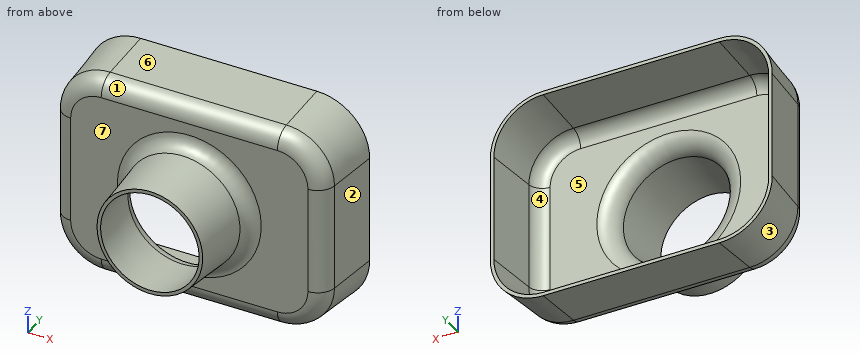
```python
from build123d import *

# Parameters (mm, degrees)
BOSS_EXTRUDE1_DEPTH = 25.4
BOSS_EXTRUDE1_DRAFT = -5
BOSS_EXTRUDE2_REACH = 83.32
SKETCH3_R           = 19.05
BOSS_EXTRUDE2_DRAFT = 5
FILLET1_R           = 5.08
FILLET2_R           = 6.35
SHELL1_T            = -1.27


with BuildPart() as part:
    # Sketch1 → Boss-Extrude1 (with draft: the straight prism first)
    with BuildSketch(Plane(origin=(0, 0, 0), x_dir=(1, 0, 0), z_dir=(0, 1, 0))):
        with BuildLine():
            ThreePointArc((31.75, -38.1), (45.220384182, -32.520384182), (50.8, -19.05))
            Line((50.8, -19.05), (50.8, 19.05))
            ThreePointArc((50.8, 19.05), (45.220384182, 32.520384182), (31.75, 38.1))
            Line((31.75, 38.1), (-31.75, 38.1))
            ThreePointArc((-31.75, 38.1), (-45.220384182, 32.520384182), (-50.8, 19.05))
            Line((-50.8, 19.05), (-50.8, -19.05))
            ThreePointArc((-50.8, -19.05), (-45.220384182, -32.520384182), (-31.75, -38.1))
            Line((-31.75, -38.1), (31.75, -38.1))
        make_face()
    extrude(amount=-BOSS_EXTRUDE1_DEPTH)
    # Boss-Extrude1: the draft: its side faces are tilted about the plane it starts from
    boss_extrude1_sides = [part.faces().sort_by_distance(p)[0] for p in [
        (45.220384182, -12.7, 32.520384182),
        (50.8, -12.7, 0),
        (45.220384182, -12.7, -32.520384182),
        (0, -12.7, -38.1),
        (-45.220384182, -12.7, -32.520384182),
        (-50.8, -12.7, 0),
        (-45.220384182, -12.7, 32.520384182),
        (0, -12.7, 38.1),
    ]]
    draft(boss_extrude1_sides, Plane(origin=(0, 0, 0), x_dir=(1, 0, 0), z_dir=(0, 1, 0)), BOSS_EXTRUDE1_DRAFT)




with BuildPart() as boss_extrude2_long_prism_1:
    # Sketch3 → Boss-Extrude2 (the long prism of profile 1, to be tilted and cut off)
    with BuildSketch(Plane(origin=(0, -50.8, 0), x_dir=(-1, 0, 0), z_dir=(0, -1, 0))):
        Circle(SKETCH3_R)
    extrude(amount=-BOSS_EXTRUDE2_REACH)
    boss_extrude2_tool1_sides = [boss_extrude2_long_prism_1.faces().sort_by_distance(p)[0] for p in [
        (19.05, -9.14, 0),
    ]]
    draft(boss_extrude2_tool1_sides, Plane(origin=(0, -50.8, 0), x_dir=(-1, 0, 0), z_dir=(0, -1, 0)), BOSS_EXTRUDE2_DRAFT)  # the draft: side faces tilted about the start plane


with BuildPart() as part_1:
    add(part.part)
    boss_extrude2_tool1 = boss_extrude2_long_prism_1.part - part.part
    add(boss_extrude2_tool1.solids().sort_by_distance((0, -50.8, 0))[0])

    # Fillet1
    fillet1_edges = [part_1.edges().sort_by_distance(p)[0] for p in [
        (21.272212054, -25.4, 0),
    ]]
    fillet(fillet1_edges, radius=FILLET1_R)

    # Fillet2
    fillet2_edges = [part_1.edges().sort_by_distance(p)[0] for p in [
        (-43.649042969, -25.4, 30.949042969),
        (0, -25.4, 35.877787946),
        (43.649042969, -25.4, 30.949042969),
        (48.577787946, -25.4, 0),
        (43.649042969, -25.4, -30.949042969),
        (0, -25.4, -35.877787946),
        (-43.649042969, -25.4, -30.949042969),
        (-48.577787946, -25.4, 0),
    ]]
    fillet(fillet2_edges, radius=FILLET2_R)

    # Shell1
    shell1_openings = [part_1.faces().sort_by_distance(p)[0] for p in [
        (0, -50.8, 0),
        (0, 0, 0),
    ]]
    offset(amount=SHELL1_T, openings=shell1_openings, kind=Kind.INTERSECTION)


solid = part_1.part
```
Input: part model. Units: mm. Frame: model coordinates. Face numbers are marked on the shaded views. A direction names the side the tool comes from. Give positions to 0.01 mm unless a question says otherwise; leave off trailing zeros. Order: outer loops, then holes, each group sorted by start corner. A loop starts at its lowest first (then second) coordinate and runs counter-clockwise, first axis right, second up. Notation, with made-up numbers: M -2.5,-33.75 L 1.5,-33.75 A33 cw 1.5,2.25 Z; hole C 0.5,88.25 d5. An arc over 180 degrees is marked long. Return JSON: item names as keys, results as strings.
Item 1: Ray query, probe 1 along X at (y, z) = (-21, -24.5); probe 2 along X at (y, z) = (-46, -1); probe 3 along Z at (x, y) = (-38.5, -3.5). Return the intervals inside material, ascending.
Solutions:
{"probe 1": "-47.91 to -46.47, 46.47 to 47.91", "probe 2": "-19.44 to -18.17, 18.17 to 19.44", "probe 3": "-36.54 to -35.16, 35.16 to 36.54"}
Item 2: Cut plane D-D (y = -16). Return loops of the section in (x, z).
Solutions:
{"outline": "M -49.4,-19.05 A17.65 ccw -31.75,-36.7 L 31.75,-36.7 A17.65 ccw 49.4,-19.05 L 49.4,19.05 A17.65 ccw 31.75,36.7 L -31.75,36.7 A17.65 ccw -49.4,19.05 Z; hole M -48.13,-19.05 A16.38 ccw -31.75,-35.43 L 31.75,-35.43 A16.38 ccw 48.13,-19.05 L 48.13,19.05 A16.38 ccw 31.75,35.43 L -31.75,35.43 A16.38 ccw -48.13,19.05 Z"}
Item 3: Pull-direction query (X, two-part tool) for the marked faces 1, 2, 3 and 4; classes: +X half, -X half, draft (parallel to the pull), parting line (faces both ways), or undercut.
Solutions:
{"face 1": "draft", "face 2": "+X half", "face 3": "-X half", "face 4": "undercut"}
Item 4: First-contact query: P1, Ø10, axis at x = -11, y = -21.5, coming from the +Z side; P2, Ø6, axis at x = 30.5, z = -18.5, coming from the +Y side; P3, Ø10, axis at x = -31, y = -5.5, coming from the +Z side. Flat tips, straight axial feed; report the tip coordinate or a pass-through.
Solutions:
{"P1": "z = 36.66", "P2": "y = -24.13", "P3": "z = 38.06"}
Item 5: Access query for the marked faces 5, 6 and 7. Directions: +Z, -Z, +X, -X, +Y, -Y. A direction counts if a zero-diameter tool reaches every point of the face in a straight line with its end or side. Return the directions, or none.
Solutions:
{"face 5": "+Y", "face 6": "+Z, +X, -X, -Y", "face 7": "-Y"}
Item 6: Cut plane C-C (x = 0). Return loops of the section in (y, z).
Solutions:
{"outline": "M -50.8,-19.05 L -30.04,-20.87 A5.08 cw -25.4,-25.93 L -25.4,-30.06 A6.35 ccw -19.6,-36.38 L 0,-38.1 L 0,-36.83 L -19.49,-35.12 A5.08 cw -24.13,-30.06 L -24.13,-25.93 A6.35 ccw -29.93,-19.6 L -50.8,-17.78 Z; M -50.8,17.78 L -29.93,19.6 A6.35 ccw -24.13,25.93 L -24.13,30.06 A5.08 cw -19.49,35.12 L 0,36.83 L 0,38.1 L -19.6,36.38 A6.35 ccw -25.4,30.06 L -25.4,25.93 A5.08 cw -30.04,20.87 L -50.8,19.05 Z"}
Item 7: Cut plane A-A (z = 0). Return loops of the section in (x, y).
Solutions:
{"outline": "M -50.8,0 L -49.08,-19.6 A6.35 ccw -42.76,-25.4 L -25.93,-25.4 A5.08 cw -20.87,-30.04 L -19.05,-50.8 L -17.78,-50.8 L -19.6,-29.93 A6.35 ccw -25.93,-24.13 L -42.76,-24.13 A5.08 cw -47.82,-19.49 L -49.53,0 Z; M 17.78,-50.8 L 19.05,-50.8 L 20.87,-30.04 A5.08 cw 25.93,-25.4 L 42.76,-25.4 A6.35 ccw 49.08,-19.6 L 50.8,0 L 49.53,0 L 47.82,-19.49 A5.08 cw 42.76,-24.13 L 25.93,-24.13 A6.35 ccw 19.6,-29.93 Z"}
Item 8: Cut plane B-B (y = -5). Return loops of the section in (x, z), then the cut area to 3 significant figures.
Solutions:
{"outline": "M -50.36,-19.05 A18.61 ccw -31.75,-37.66 L 31.75,-37.66 A18.61 ccw 50.36,-19.05 L 50.36,19.05 A18.61 ccw 31.75,37.66 L -31.75,37.66 A18.61 ccw -50.36,19.05 Z; hole M -49.09,-19.05 A17.34 ccw -31.75,-36.39 L 31.75,-36.39 A17.34 ccw 49.09,-19.05 L 49.09,19.05 A17.34 ccw 31.75,36.39 L -31.75,36.39 A17.34 ccw -49.09,19.05 Z", "area": "403 mm^2"}
